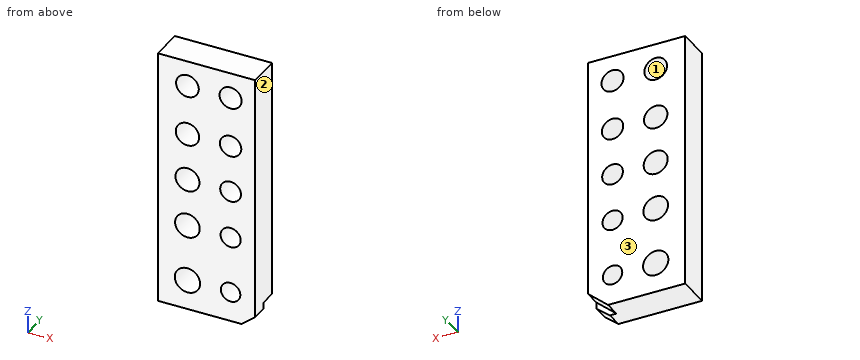
Autodesk Inventor part; units mm, degrees
ref_plane "YZ Plane" through (0, 0, 0) normal (1, 0, 0) x (0, 1, 0)
ref_plane "XZ Plane" through (0, 0, 0) normal (0, 1, 0) x (-1, 0, 0)
ref_plane "XY Plane" through (0, 0, 0) normal (0, 0, 1) x (1, 0, 0)
sketch "Sketch1" plane through (0, 0, 0) normal (0, 1, 0) x (-1, 0, 0)
  line L0 (0, 0) -> (15, 0)
  line L1 (15, 0) -> (15, 40)
  line L2 (15, 40) -> (0, 40)
  line L3 (0, 40) -> (0, 0)
  circle A0 centre (3.7979, 4.6387) radius 1.5
  circle A1 centre (3.7979, 13.4768) radius 1.55
  circle A2 centre (3.7979, 20.9025) radius 1.6
  circle A3 centre (3.7979, 28.2372) radius 1.65
  circle A4 centre (3.7979, 36.0274) radius 1.7
  circle A5 centre (10.4492, 36.0274) radius 1.75
  circle A6 centre (10.4492, 28.2372) radius 1.8
  circle A7 centre (10.4492, 20.9025) radius 1.85
  circle A8 centre (10.4492, 13.4768) radius 1.9
  circle A9 centre (10.4492, 4.6387) radius 1.95
  line L4 (2.0979, 0) -> (0, 1.698)
  point P0 (7.5, 40)
  dimension "d0" = 3
  dimension "d1" = 3.1
  dimension "d2" = 3.2
  dimension "d3" = 3.3
  dimension "d4" = 3.4
  dimension "d5" = 3.5
  dimension "d6" = 3.6
  dimension "d7" = 3.7
  dimension "d8" = 3.8
  dimension "d9" = 3.9
  dimension "d10" = 40
  dimension "d11" = 15
extrude "Extrusion1" add sketch "Sketch1" along normal blind 5 contours L4 L3 L2 L1 L0
sketch "Sketch2" plane through (0, 5, 0) normal (0, 1, 0) x (1, 0, 0)
  line L0 (0, -40) -> (0, -1.698)
  line L1 (0, -1.698) -> (-2.0979, 0)
  line L2 (-2.0979, 0) -> (0, -1.698)
  line L3 (0, -1.698) -> (0, -2.698)
  line L4 (-2.0979, 0) -> (-3.0979, 0)
  line L5 (-2.0979, 0) -> (-15, 0)
  line L6 (-3.0979, 0) -> (0, -2.698)
  point P0 (0, 0)
  dimension "d14" = 1
  dimension "d15" = 1
extrude "Extrusion2" cut sketch "Sketch2" against normal blind 2.5
properties part number "m3_sizing_tests"
Input: part model. Units: mm. Frame: model coordinates. Face numbers are marked on the shaded views. Coordinates: 2 decimals unless noted, no trailing zeros. Write each loop counter-clockwise with the first axis right and the second up, starting at its lowest first coordinate (ties: lowest second). Pieces come first, ordered by that corner, then holes.
1) Section C-C on y = 4.45. State how many separate pieces and enclosed holes the cut face has, and give its area (3 significant figures).
2) Pin query (flat end, axial travel): pin 1 Ø3 at (x, z) = (-10.45, 4.64) entering from -Y; pin 2 Ø4.5 at (x, z) = (-3.8, 36.03) entering from -Y. Return the tip coordinate at first contact, or that it passes through.
3) Mould query, pull axis X, two halves, no side actions, for the marked faces 1, 2 and 3. Classes: pulls with the +X half, pulls with the -X half, needs draft (parallel to the pull), parting line crosses it, or undercut.
4) Section B-B on z = 27. Output: boundary loops of the cut face in (x, y), and give its area (3 significant figures).
5) Material intervals for line 1 along X through (y, z) = (4.25, 20); line 2 along X through (y, z) = (1, 12.5); line 3 along Z through (x, y) = (-3.5, 1.15), sorted ascending.
6) Section D-D on x = -9.25. Output: boundary loops of the cut face in (y, z).
7) Section A-A on x = -4. Output: boundary loops of the cut face in (y, z), and give its area (3 significant figures).
Check result:
1. separate pieces: 1
1. enclosed holes: 10
1. area: 502 mm2
2. pin 1: passes through
2. pin 2: stops at y = 0
3. face 1: undercut
3. face 2: pulls with the +X half
3. face 3: needs draft
4. outline: (-15, 0) - (-11.76, 0) - (-11.76, 5) - (-15, 5) - close; (-9.14, 0) - (-4.89, 0) - (-4.89, 5) - (-9.14, 5) - close; (-2.71, 0) - (0, 0) - (0, 5) - (-2.71, 5) - close
4. area: 51.0 mm2
5. line 1: x = -15 to -12.06, -8.83 to -5.12, -2.48 to 0
5. line 2: x = -15 to -12.08, -8.82 to -5, -2.59 to 0
5. line 3: z = 0 to 3.17, 6.11 to 11.96, 15 to 19.33, 22.47 to 26.61, 29.86 to 34.35, 37.7 to 40
6. outline: (0, 0) - (5, 0) - (5, 3.1) - (0, 3.1) - close; (0, 6.18) - (5, 6.18) - (5, 12) - (0, 12) - close; (0, 14.95) - (5, 14.95) - (5, 19.49) - (0, 19.49) - close; (0, 22.31) - (5, 22.31) - (5, 26.89) - (0, 26.89) - close; (0, 29.58) - (5, 29.58) - (5, 34.75) - (0, 34.75) - close; (0, 37.3) - (5, 37.3) - (5, 40) - (0, 40) - close
7. outline: (0, 0) - (5, 0) - (5, 3.15) - (0, 3.15) - close; (0, 6.13) - (5, 6.13) - (5, 11.94) - (0, 11.94) - close; (0, 15.01) - (5, 15.01) - (5, 19.32) - (0, 19.32) - close; (0, 22.49) - (5, 22.49) - (5, 26.6) - (0, 26.6) - close; (0, 29.87) - (5, 29.87) - (5, 34.34) - (0, 34.34) - close; (0, 37.72) - (5, 37.72) - (5, 40) - (0, 40) - close
7. area: 121 mm2
